Drawing for the job (mm, zero at the part's lowest x, y, z). A direction names the side the tool comes from. Coordinates: 2 decimals unless noted, no trailing zeros. Loops run counter-clockwise (first coordinate to the right, second up) from the corner with the lowest first, then second, coordinate; pieces in that order, holes last. Notation, with made-up numbers: (-11.5, 80) - (36.5, 80) arc R12 ccw to (36.5, 102) - close; hole circle Ø3 at (-2.5, 5.25). An arc over 180 degrees is marked (long way). Put each result on its own line as item: value.
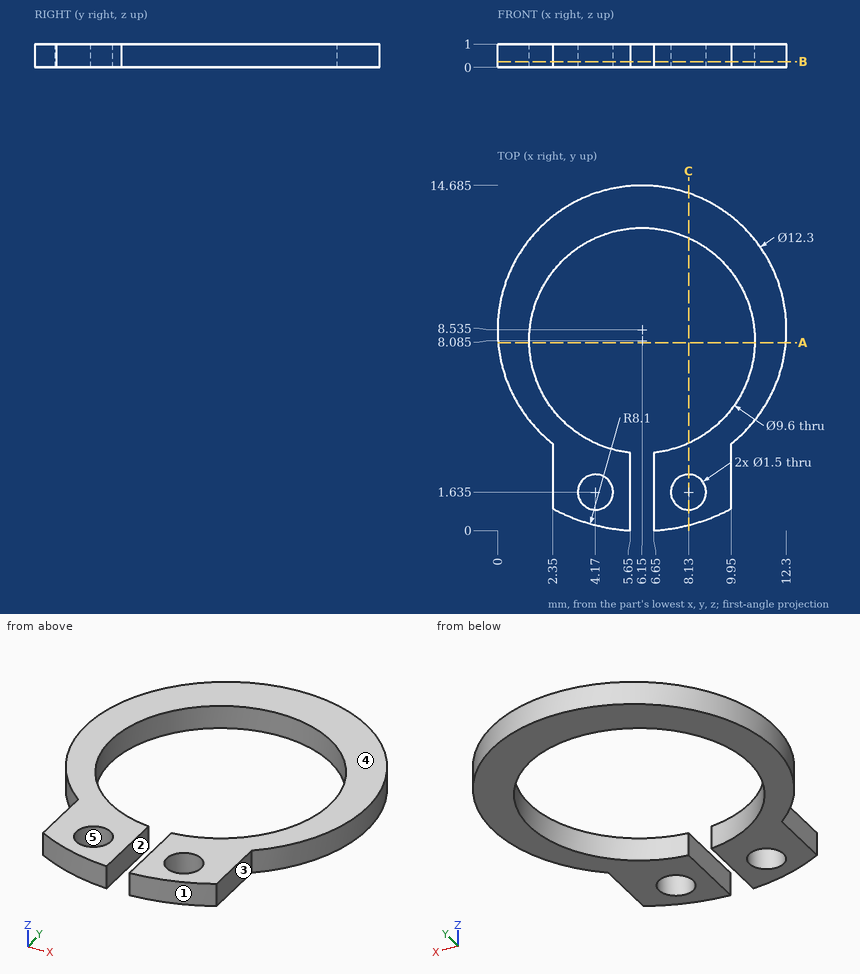
Q1. Tool access for the marked faces 1 and 2: list every direction of +Z, -Z, +X, -X, +Y, -Y with a clear straight run to the whole face (end or side of a thin tool).
Determined:
face 1: +Z, -Z, +X, -Y
face 2: +Z, -Z, -Y
Q2. Wall check: L1, parallel to X at y = 1.5, z = 0.85; L2, parallel to Y at x = 4.17, z = 0.55 (1 decimal); L3, parallel to Y at x = 4, z = 0.4 (1 decimal). Give the ranges that are in metal, low to high. Write a range as from..to.
Determined:
L1: 2.35..3.43, 4.91..5.65, 6.65..7.39, 8.87..9.95
L2: 0.2..0.9, 2.4..3.7, 12.5..14.4
L3: 0.3..0.9, 2.4..3.8, 12.4..14.3
Q3. Pin check, flat tips, straight feed: pin 1 Ø6 at (x, y) = (8, 9.5) entering from +Z; pin 2 Ø0.9 at (x, y) = (4.17, 1.63) entering from -Z. Stop position of each tip, or through.
Determined:
pin 1: z = 1
pin 2: through
Q4. Mould opens along X. For the marked faces 3, 4 and 5 say: +X half, -X half, draft (parallel to the pull), parting line (faces both ways), or undercut.
Determined:
face 3: +X half
face 4: draft
face 5: undercut
Q5. Slice it at A-A, the plane y = 8. Give the cut face in (x, z).
Determined:
outline: (0.02, 0) - (1.35, 0) - (1.35, 1) - (0.02, 1) - close; (10.95, 0) - (12.28, 0) - (12.28, 1) - (10.95, 1) - close
Q6. Slice it at B-B, the plane z = 0.25. State how many separate pieces and enclosed holes the cut face has.
Determined:
separate pieces: 1
enclosed holes: 2
Q7. Slice it at C-C, the plane x = 8.13. Give the cut face in (y, z) (1 decimal).
Determined:
outline: (0.2, 0) - (0.9, 0) - (0.9, 1) - (0.2, 1) - close; (2.4, 0) - (3.7, 0) - (3.7, 1) - (2.4, 1) - close; (12.5, 0) - (14.4, 0) - (14.4, 1) - (12.5, 1) - close
